```python
from build123d import *

# Parameters (mm, degrees)
SKETCH1_R           = 12.427436065
BOSS_EXTRUDE1_DEPTH = 5
CUT_EXTRUDE1_DEPTH  = 4
CUT_EXTRUDE2_DEPTH  = 6


with BuildPart() as part:
    # Sketch1 → Boss-Extrude1 (new body)
    with BuildSketch(Plane(origin=(0, 0, 0), x_dir=(1, 0, 0), z_dir=(0, 1, 0))):
        with Locations((-0.572563935, 0)):
            Circle(SKETCH1_R)
        with BuildLine():
            ThreePointArc((-9.837575138, 1.742446029), (-9.678767906, 2.44), (-9.467522018, 3.123503075))
            ThreePointArc((-9.467522018, 3.123503075), (-7.221418603, 3.838718032), (-7.725075989, 6.141508127))
            ThreePointArc((-7.725075989, 6.141508127), (-7.238767906, 6.66620397), (-6.714072063, 7.152512053))
            ThreePointArc((-6.714072063, 7.152512053), (-4.411281968, 6.648854668), (-3.696067011, 8.894958082))
            ThreePointArc((-3.696067011, 8.894958082), (-3.012563935, 9.10620397), (-2.315009965, 9.265011203))
            ThreePointArc((-2.315009965, 9.265011203), (-0.572563935, 7.677436065), (1.169882094, 9.265011203))
            ThreePointArc((1.169882094, 9.265011203), (1.867436065, 9.10620397), (2.55093914, 8.894958082))
            ThreePointArc((2.55093914, 8.894958082), (3.266154097, 6.648854668), (5.568944192, 7.152512053))
            ThreePointArc((5.568944192, 7.152512053), (6.093640035, 6.66620397), (6.579948118, 6.141508127))
            ThreePointArc((6.579948118, 6.141508127), (6.076290732, 3.838718032), (8.322394147, 3.123503075))
            ThreePointArc((8.322394147, 3.123503075), (8.533640035, 2.44), (8.692447267, 1.742446029))
            ThreePointArc((8.692447267, 1.742446029), (7.104872129, 0), (8.692447267, -1.742446029))
            ThreePointArc((8.692447267, -1.742446029), (8.533640035, -2.44), (8.322394147, -3.123503075))
            ThreePointArc((8.322394147, -3.123503075), (6.076290732, -3.838718032), (6.579948118, -6.141508127))
            ThreePointArc((6.579948118, -6.141508127), (6.093640035, -6.66620397), (5.568944192, -7.152512053))
            ThreePointArc((5.568944192, -7.152512053), (3.266154097, -6.648854668), (2.55093914, -8.894958082))
            ThreePointArc((2.55093914, -8.894958082), (1.867436065, -9.10620397), (1.169882094, -9.265011203))
            ThreePointArc((1.169882094, -9.265011203), (-0.572563935, -7.677436065), (-2.315009965, -9.265011203))
            ThreePointArc((-2.315009965, -9.265011203), (-3.012563935, -9.10620397), (-3.696067011, -8.894958082))
            ThreePointArc((-3.696067011, -8.894958082), (-4.411281968, -6.648854668), (-6.714072063, -7.152512053))
            ThreePointArc((-6.714072063, -7.152512053), (-7.238767906, -6.66620397), (-7.725075989, -6.141508127))
            ThreePointArc((-7.725075989, -6.141508127), (-7.221418603, -3.838718032), (-9.467522018, -3.123503075))
            ThreePointArc((-9.467522018, -3.123503075), (-9.678767906, -2.44), (-9.837575138, -1.742446029))
            ThreePointArc((-9.837575138, -1.742446029), (-8.25, 0), (-9.837575138, 1.742446029))
        make_face(mode=Mode.SUBTRACT)
    extrude(amount=BOSS_EXTRUDE1_DEPTH)

    # Sketch3 → Cut-Extrude1 (cut)
    with BuildSketch(Plane(origin=(0, 5, 0), x_dir=(1, 0, 0), z_dir=(0, 1, 0))):
        with BuildLine():
            ThreePointArc((6.169043579, -7.287298192), (4.053237314, -8.783845947), (1.622190338, -9.681789116))
            Line((1.622190338, -9.681789116), (2.17488951, -12.119928494))
            ThreePointArc((2.17488951, -12.119928494), (5.218140623, -10.995858668), (7.866764791, -9.122439246))
            Line((7.866764791, -9.122439246), (6.169043579, -7.287298192))
        make_face()
        with BuildLine():
            Line((2.17488951, -12.119928494), (1.622190338, -9.681789116))
            ThreePointArc((1.622190338, -9.681789116), (-8.329569464, 6.19538958), (9.354872129, 0))
            ThreePointArc((9.354872129, 0), (8.523612855, -3.976626035), (6.169043579, -7.287298192))
            Line((6.169043579, -7.287298192), (7.866764791, -9.122439246))
            ThreePointArc((7.866764791, -9.122439246), (10.814279027, -4.978049265), (11.854872129, 0))
            ThreePointArc((11.854872129, 0), (-10.282995676, 7.755558172), (2.17488951, -12.119928494))
        make_face()
    extrude(amount=-CUT_EXTRUDE1_DEPTH, mode=Mode.SUBTRACT)

    # Sketch3<3> → Cut-Extrude2 (cut, through all)
    with BuildSketch(Plane(origin=(0, 5, 0), x_dir=(1, 0, 0), z_dir=(0, 1, 0))):
        Polygon((55.39886132, -60.501959687), (7.866764791, -9.122439246), (-0.572563935, 0), (2.17488951, -12.119928494), (17.649132378, -80.381946696), (82.878094772, -204.24398184), (120.627823714, -184.363994832), align=None)
    extrude(amount=-CUT_EXTRUDE2_DEPTH, mode=Mode.SUBTRACT)


solid = part.part
```
CAD build for the part. Positions are in the model's coordinates, mm. A direction names the side the tool comes from. Round coordinates to 2 decimals unless told otherwise and drop trailing zeros. Order: outer loops, then holes, each group sorted by start corner. A loop starts at its lowest first (then second) coordinate and runs counter-clockwise, first axis right, second up.
Q1. Slice it at D-D (z = 10.75). Write the cut outline in (x, y), and give its area (3 significant figures).
Q2. Two-plate mould, pull along Z, no slides. Class faces 1 (the cylindrical face through (7.105, 2.465, -0.036)), 2 (the flat face through (6.55, 0.84, 7.7)), 3 (the flat face through (-1, 0, -8)): pulls with the +Z half, pulls with the -Z half, needs draft (parallel to the pull), parting line crosses it, or undercut.
Q3. Slice it at A-A (z = 5). Write the cut outline in (x, y).
Q4. Drop flat-ended pins along their axis: pin 1 (3 mm diameter, centred on x = -6, z = 6.5, fed in from -Y); pin 2 (8 mm diameter, centred on x = -4, z = 1, fed in from -Y); pin 3 (2 mm diameter, centred on x = 3, y = 2.5, fed in from +Z). Give the stop position or say it passes through.
Q5. Which spindle directions (+Z, -Z, +X, -X, +Y, -Y) get a long thin tool onto all of the face, cutting with end or side? Do faces 4 (the cylindrical face through (1.86, 2.46, -9.11)), 5 (the flat face through (-5, 5, -7)). Say none if no direction does.
Q6. Wall check: L1, parallel to Y at x = -3.75, z = 11.25; L2, parallel to Z at x = -2.5, y = 2.3; L3, parallel to X at y = 1.1, z = -3.25. Give the ranges that are in metal, low to high.
Q7. Slice it at B-B (x = -6). Write the cut outline in (y, z).
Results below:
1. outline: (-6.81, 0) - (1.86, 0) - (1.86, 1) - (-6.81, 1) - close
1. area: 8.67 mm2
2. face 1: undercut
2. face 2: pulls with the +Z half
2. face 3: needs draft
3. outline: (-11.95, 0) - (-7.01, 0) - (-7.01, 5) - (-9.15, 5) - (-9.15, 1) - (-11.95, 1) - close; (5.87, 0) - (10.8, 0) - (10.8, 1) - (8, 1) - (8, 5) - (5.87, 5) - close
4. pin 1: stops at y = 0
4. pin 2: passes through
4. pin 3: stops at z = -6.42
5. face 4: +Y, -Y
5. face 5: +Z, -Z, +X, -X, +Y
6. L1: y = 0 to 1
6. L2: z = -9.74 to -9.23, 9.23 to 9.74
6. L3: x = -9.95 to -7.78, 6.63 to 8.81
7. outline: (0, -11.18) - (1, -11.18) - (1, -8.31) - (5, -8.31) - (5, -6.57) - (0, -6.57) - close; (0, 6.57) - (5, 6.57) - (5, 8.31) - (1, 8.31) - (1, 11.18) - (0, 11.18) - close
